The model under review builds one solid part; all positions refer to its coordinate system, in mm. A direction names the side the tool comes from. Give positions to 0.01 mm unless a question says otherwise; leave off trailing zeros. Write each loop counter-clockwise with the first axis right and the second up, starting at its lowest first coordinate (ties: lowest second). Pieces come first, ordered by that corner, then holes. Notation, with made-up numbers: (-39, 14.5) -> (14, 14.5) arc R26 ccw to (14, 35.5) -> close; hole circle Ø4 at (47, 67). An arc over 180 degrees is marked (long way). Use CSV: the item, a comma, the result in double quotes.
```python
from build123d import *

# Parameters (mm, degrees)
SKETCH_1_R                   = 85
EXTRUDE_1_DEPTH              = 5
HOLE_WIZARD_M3_1_D           = 3
HOLE_WIZARD_M3_1_CSINK_D     = 6.72
HOLE_WIZARD_M3_1_CSINK_ANGLE = 90
SKETCH_3_R                   = 25
SKETCH_3_R_2                 = 23
CUT_EXTRUDE_2_DEPTH          = 5
SKETCH_14_R                  = 30.8
SKETCH_14_R_2                = 28
CUT_EXTRUDE_5_DEPTH          = 1.5
FILLET_1_R                   = 1
HOLE_WIZARD_M2_5_3_D         = 2.5
HOLE_WIZARD_M2_5_3_DEPTH     = 3
HOLE_WIZARD_M2_5_3_TIP       = 0.751075774
HOLE_WIZARD_M3_2_D           = 2.5


with BuildPart() as part:
    # 草图1 → 凸台-拉伸1 (new body)
    with BuildSketch(Plane(origin=(0, 0, 0), x_dir=(1, 0, 0), z_dir=(0, 1, 0))):
        with Locations(Location((0, 0, 0), (0, 0, 270))):
            Circle(SKETCH_1_R)
    extrude(amount=EXTRUDE_1_DEPTH)

    # M3 螺纹孔1 (through all)
    with Locations(Plane(origin=(0, 5, -80), x_dir=(0, 0, 1), z_dir=(0, 1, 0))):
        with Locations((0, 0), (23.431457505, 56.568542495), (80, 80), (136.568542495, 56.568542495), (160, 0), (136.568542495, -56.568542495), (23.431457505, -56.568542495), (80, -80)):
            CounterSinkHole(HOLE_WIZARD_M3_1_D / 2, HOLE_WIZARD_M3_1_CSINK_D / 2, counter_sink_angle=HOLE_WIZARD_M3_1_CSINK_ANGLE)

    # 草图3 → 切除-拉伸2 (cut)
    with BuildSketch(Plane(origin=(0, 5, 0), x_dir=(1, 0, 0), z_dir=(0, 1, 0))):
        with Locations(Location((-20, 0, 0), (0, 0, 270))):
            Circle(SKETCH_3_R)
        with Locations(Location((42, 0, 0), (0, 0, 270))):
            Circle(SKETCH_3_R_2)
    extrude(amount=-CUT_EXTRUDE_2_DEPTH, mode=Mode.SUBTRACT)

    # 草图6 → 旋转1 (revolve)
    with BuildSketch(Plane.XY, mode=Mode.PRIVATE) as revolve_1_sk:
        Polygon((19, 5), (29.5, -8), (36.7, -8), (36.7, -9), (39, -9), (39, -10), (27.5, -10), (19, 0), align=None)
    revolve(revolve_1_sk.sketch.rotate(Axis((42, 0, 0), (0, -1, 0)), 270), axis=Axis((42, 0, 0), (0, -1, 0)))

    # 草图14 → 切除-拉伸5 (cut)
    with BuildSketch(Plane(origin=(0, 5, 0), x_dir=(1, 0, 0), z_dir=(0, 1, 0))):
        with Locations(Location((-20, 0, 0), (0, 0, 270))):
            Circle(SKETCH_14_R)
        with Locations(Location((-20, 0, 0), (0, 0, 270))):
            Circle(SKETCH_14_R_2, mode=Mode.SUBTRACT)
    extrude(amount=-CUT_EXTRUDE_5_DEPTH, mode=Mode.SUBTRACT)

    # 圆角1
    fillet_1_edges = [part.edges().sort_by_distance(p)[0] for p in [
        (0, 5, -85),
    ]]
    fillet(fillet_1_edges, radius=FILLET_1_R)

    # M2.5 螺纹孔3
    with Locations(Plane(origin=(-20, 5, -32.5), x_dir=(0, 0, 1), z_dir=(0, 1, 0))):
        with Locations((0, 0), (16.25, 28.145825623), (48.75, 28.145825623), (65, 0), (16.25, -28.145825623), (48.75, -28.145825623)):
            Hole(HOLE_WIZARD_M2_5_3_D / 2, depth=HOLE_WIZARD_M2_5_3_DEPTH)
            with Locations((0, 0, -(HOLE_WIZARD_M2_5_3_DEPTH + HOLE_WIZARD_M2_5_3_TIP / 2))):  # 118° drill point
                Cone(0, HOLE_WIZARD_M2_5_3_D / 2, HOLE_WIZARD_M2_5_3_TIP, mode=Mode.SUBTRACT)

    # M3 螺纹孔2 (through all)
    with Locations(Plane(origin=(-73.910362601, 5, 30.614674589), x_dir=(0, 0, 1), z_dir=(0, 1, 0))):
        with Locations((0, 0), (-61.229349178, 147.820725202)):
            Hole(HOLE_WIZARD_M3_2_D / 2)


solid = part.part
```
Q1. Consider section A-A (y = -6). Write out the cut boundary in (x, z), then the cut area to 3 significant figures.
Derived:
outline,"circle Ø35.8 at (42, 0); hole circle Ø28.23 at (42, 0)"
area,"381 mm2"
Q2. The part is to be moulded in two halves that separate along Z. For faces 3 (the conical face through (37.48, -9.37, 14.34)), 4 (the cylindrical face through (37.5, -8.5, 2.8)), 5 (the flat face through (20, 5, 17)), say which applies: pulls with the +Z half, pulls with the -Z half, needs draft (parallel to the pull), parting line crosses it, or undercut.
Derived:
face 3,"parting line crosses it"
face 4,"undercut"
face 5,"needs draft"
Q3. To check wall thickness, follow probe 1 along X at (y, z) = (4.05, 32.5); probe 2 along X at (y, z) = (2.3, 0); probe 3 along X at (y, z) = (0.75, -0.5) (3 decimals). State the ranges of each line that lie inside material, in increasing order.
Derived:
probe 1,"x = -78.54 to -21.25, -18.75 to 78.54"
probe 2,"x = -85 to -81.5, -78.5 to -45, 5 to 21.18, 62.82 to 78.5, 81.5 to 85"
probe 3,"x = -84.999 to -81.414, -78.586 to -44.995, 4.995 to 22.439, 61.561 to 78.586, 81.414 to 84.999"
Q4. Insertion check: pin 1 (7.5 mm diameter, centred on x = 42, z = -2.5, fed in from +Y); pin 2 (1.5 mm diameter, centred on x = -48.15, z = -16.25, fed in from -Y); pin 3 (2 mm diameter, centred on x = 73.91, z = -30.61, fed in from -Y); pin 4 (4 mm diameter, centred on x = 56.57, z = -56.57, fed in from +Y). Each pin has a flat end and moves straight along its axis. Give the tip position at first contact, or say it passes through.
Derived:
pin 1,"stops at y = -8"
pin 2,"stops at y = 0"
pin 3,"passes through"
pin 4,"stops at y = 3.64"
Q5. Machinability: for faces 1 (the cylindrical face through (-51.721, 1.972, -67.453)), 2 (the flat face through (45, -8, 5)), which of the approach directions +Z, -Z, +X, -X, +Y, -Y give a long, thin tool a straight path to every point of the face, cutting with its end or side? Answer none if there is none.
Derived:
face 1,"+Y, -Y"
face 2,"+Y"
